```python
from build123d import *


with BuildPart() as part:
    # Sweep1: sweep along a path in Sketch2
    with BuildLine(Plane.XY) as sweep1_path:
        Line((2.459788124, -32.166085282), (-149.640466326, -43.797416737))
        ThreePointArc((-149.640466326, -43.797416737), (-167.230963528, -27.339263039), (-149.320184824, -11.230246272))
        Line((-149.320184824, -11.230246272), (-58.083261257, -20.015194383))
        ThreePointArc((-58.083261257, -20.015194383), (-52.202583099, -18.950464372), (-47.746530099, -14.968050876))
        Line((-47.746530099, -14.968050876), (-27.222888137, 17.309591604))
        ThreePointArc((-27.222888137, 17.309591604), (27.663395153, 16.596510736), (2.459788124, -32.166085282))
    # Sketch3 → Sweep1 (sweep)
    with BuildSketch(Plane(origin=(0, 0, 0), x_dir=(1, 0, 0), z_dir=(0, 1, 0))):
        Polygon((32.26, 0), (32.26, -4.5), (33.26, -4.5), (33.26, 4.5), (32.26, 4.5), align=None)
    sweep(path=sweep1_path.line)


solid = part.part
```
Input: part model. Units: mm. Frame: model coordinates. A direction names the side the tool comes from. Give positions to 0.01 mm unless a question says otherwise; leave off trailing zeros. Order: outer loops, then holes, each group sorted by start corner. A loop starts at its lowest first (then second) coordinate and runs counter-clockwise, first axis right, second up. Notation, with made-up numbers: (13.5, 37.5) - (45.5, 37.5) arc R13 cw to (45.5, 59.5) - close; hole circle Ø11 at (70, 77.5). An arc over 180 degrees is marked (long way). Put each result on its own line as item: value.
Item 1: Section query C-C, the plane y = 0. Return loops of the section in (x, z).
Found:
outline: (-39.41, -4.5) - (-38.23, -4.5) - (-38.23, 4.5) - (-39.41, 4.5) - close; (32.26, -4.5) - (33.26, -4.5) - (33.26, 4.5) - (32.26, 4.5) - close
Item 2: Ray query, L1, parallel to X at y = 0, z = -0.75; L2, parallel to Y at x = 0, z = -2.5; L3, parallel to Y at x = -79.5, z = 0. Return the intervals inside material, ascending. Write a range as from..to.
Found:
L1: x = -39.41..-38.23, 32.26..33.26
L2: y = -33.36..-32.35, 32.26..33.26
L3: y = -39.44..-38.43, -17.95..-16.95
Item 3: Access query for faces 1 (the flat face through (-37.34, 1.4, -0.06)), 2 (the cylindrical face through (-52.711, -18.085, -0.063)). Directions: +Z, -Z, +X, -X, +Y, -Y. A direction counts if a zero-diameter tool reaches every point of the face in a straight line with its end or side. Return the directions, or none.
Found:
face 1: +Z, -Z
face 2: +Z, -Z, +Y
Item 4: Section query A-A, the plane y = -38.5. Return loops of the section in (x, z), then the cut area to 3 significant figures.
Found:
outline: (-164.3, -4.5) - (-162.98, -4.5) - (-162.98, 4.5) - (-164.3, 4.5) - close; (-80.37, -4.5) - (-67.25, -4.5) - (-67.25, 4.5) - (-80.37, 4.5) - close
area: 130 mm^2
Item 5: Section query B-B, the plane z = 1. Return loops of the section in (x, y) (1 decimal).
Found:
outline: (-149.6, -44.8) - (2.5, -33.2) arc R33.3 ccw (long way) to (-28.1, 17.8) - (-48.6, -14.4) arc R10 cw to (-58, -19) - (-149.2, -10.2) arc R17.3 ccw (long way) to start; hole (-149.6, -43.8) - (2.5, -32.2) arc R32.3 ccw (long way) to (-27.2, 17.3) - (-47.7, -15) arc R11 cw to (-58.1, -20) - (-149.3, -11.2) arc R16.3 ccw (long way) to start
Item 6: Draft query along X for faces 3 (the flat face through (-74.58, -39.06, 0.06)), 4 (the flat face through (-102.97, -14.69, 0.06)), 5 (the flat face through (-46, -11, -4.5)). Return one class per face: +X half, -X half, draft (parallel to the pull), parting line (faces both ways), or undercut.
Found:
face 3: +X half
face 4: undercut
face 5: draft
Item 7: Contact query for flat-ended pins moving along their axis: pin 1 (3 mm diameter, centred on x = -61.5, z = 0.5, fed in from +Y); pin 2 (1 mm diameter, centred on x = -133, z = -2.5, fed in from -Y). Output: stop coordinate, or through.
Found:
pin 1: stops at y = -18.54
pin 2: stops at y = -43.57
